from build123d import *

# Parameters (mm, degrees)
SKETCH1_R                  = 54.76875
BOSS_EXTRUDE1_DEPTH        = 6.35
BOSS_EXTRUDE2_START        = -6.35
BOSS_EXTRUDE2_DEPTH        = 6.35
F_1_0_228_DIAMETER_HOLE1_D = 5.7912
SKETCH11_R                 = 1.5875
CUT_EXTRUDE1_DEPTH         = 3.175
SKETCH12_R                 = 23.8125
CUT_EXTRUDE2_DEPTH         = 92.146558235


with BuildPart() as part:
    # Sketch1 → Boss-Extrude1 (new body)
    with BuildSketch(Plane.XY):
        Circle(SKETCH1_R)
    extrude(amount=BOSS_EXTRUDE1_DEPTH)

    # Sketch7 → Boss-Extrude2 (add)
    with BuildSketch(Plane.XY.offset(6.35).offset(BOSS_EXTRUDE2_START)):
        with BuildLine():
            Line((-54.561291868, 4.7625), (-59.53125, 4.7625))
            ThreePointArc((-59.53125, 4.7625), (-64.29375, 0), (-59.53125, -4.7625))
            Line((-59.53125, -4.7625), (-54.561291868, -4.7625))
            ThreePointArc((-54.561291868, -4.7625), (-54.76875, 0), (-54.561291868, 4.7625))
        make_face()
        with BuildLine():
            Line((-4.7625, 59.53125), (-4.7625, 54.561291868))
            ThreePointArc((-4.7625, 54.561291868), (0, 54.76875), (4.7625, 54.561291868))
            Line((4.7625, 54.561291868), (4.7625, 59.53125))
            ThreePointArc((4.7625, 59.53125), (0, 64.29375), (-4.7625, 59.53125))
        make_face()
        with BuildLine():
            ThreePointArc((4.7625, -54.561291868), (0, -54.76875), (-4.7625, -54.561291868))
            Line((-4.7625, -54.561291868), (-4.7625, -59.53125))
            ThreePointArc((-4.7625, -59.53125), (0, -64.29375), (4.7625, -59.53125))
            Line((4.7625, -59.53125), (4.7625, -54.561291868))
        make_face()
        with BuildLine():
            Line((59.53125, 4.7625), (54.561291868, 4.7625))
            ThreePointArc((54.561291868, 4.7625), (54.76875, 0), (54.561291868, -4.7625))
            Line((54.561291868, -4.7625), (59.53125, -4.7625))
            ThreePointArc((59.53125, -4.7625), (64.29375, 0), (59.53125, 4.7625))
        make_face()
    extrude(amount=BOSS_EXTRUDE2_DEPTH)

    # #1 (0.228) Diameter Hole1 (through all)
    with Locations(Plane.XY.offset(6.35)):
        with Locations((-59.53125, 0), (0, 59.53125), (59.53125, 0), (0, -59.53125)):
            Hole(F_1_0_228_DIAMETER_HOLE1_D / 2)

    # Sketch11 → Cut-Extrude1 (cut)
    with BuildSketch(Plane.XY.offset(6.35)):
        with Locations((-47.625, 0)):
            Circle(SKETCH11_R)
        with Locations((-46.584279485, 9.901794275)):
            Circle(SKETCH11_R)
        with Locations((-43.50760242, 19.370832626)):
            Circle(SKETCH11_R)
        with Locations((-38.529434357, 27.99327264)):
            Circle(SKETCH11_R)
        with Locations((-31.867345128, 35.392272313)):
            Circle(SKETCH11_R)
        with Locations((-23.8125, 41.244459855)):
            Circle(SKETCH11_R)
        with Locations((-14.716934357, 45.294066589)):
            Circle(SKETCH11_R)
        with Locations((-4.978168063, 47.364105267)):
            Circle(SKETCH11_R)
        with Locations((4.978168063, 47.364105267)):
            Circle(SKETCH11_R)
        with Locations((14.716934357, 45.294066589)):
            Circle(SKETCH11_R)
        with Locations((23.8125, 41.244459855)):
            Circle(SKETCH11_R)
        with Locations((31.867345128, 35.392272313)):
            Circle(SKETCH11_R)
        with Locations((38.529434357, 27.99327264)):
            Circle(SKETCH11_R)
        with Locations((43.50760242, 19.370832626)):
            Circle(SKETCH11_R)
        with Locations((46.584279485, 9.901794275)):
            Circle(SKETCH11_R)
        with Locations((47.625, 0)):
            Circle(SKETCH11_R)
        with Locations((46.584279485, -9.901794275)):
            Circle(SKETCH11_R)
        with Locations((43.50760242, -19.370832626)):
            Circle(SKETCH11_R)
        with Locations((38.529434357, -27.99327264)):
            Circle(SKETCH11_R)
        with Locations((31.867345128, -35.392272313)):
            Circle(SKETCH11_R)
        with Locations((23.8125, -41.244459855)):
            Circle(SKETCH11_R)
        with Locations((14.716934357, -45.294066589)):
            Circle(SKETCH11_R)
        with Locations((4.978168063, -47.364105267)):
            Circle(SKETCH11_R)
        with Locations((-4.978168063, -47.364105267)):
            Circle(SKETCH11_R)
        with Locations((-14.716934357, -45.294066589)):
            Circle(SKETCH11_R)
        with Locations((-23.8125, -41.244459855)):
            Circle(SKETCH11_R)
        with Locations((-31.867345128, -35.392272313)):
            Circle(SKETCH11_R)
        with Locations((-38.529434357, -27.99327264)):
            Circle(SKETCH11_R)
        with Locations((-43.50760242, -19.370832626)):
            Circle(SKETCH11_R)
        with Locations((-46.584279485, -9.901794275)):
            Circle(SKETCH11_R)
    extrude(amount=-CUT_EXTRUDE1_DEPTH, mode=Mode.SUBTRACT)

    # Sketch12 → Cut-Extrude2 (cut, through all)
    with BuildSketch(Plane.XY.offset(6.35)):
        Circle(SKETCH12_R)
    extrude(amount=-CUT_EXTRUDE2_DEPTH, mode=Mode.SUBTRACT)


solid = part.part
Design review of the part built by this model. Coordinates are the model's own, in mm. A direction names the side the tool comes from. Coordinates: 2 decimals unless noted, no trailing zeros. Order: outer loops, then holes, each group sorted by start corner. A loop starts at its lowest first (then second) coordinate and runs counter-clockwise, first axis right, second up.
Item 1: Take a section at C-C, the plane z = 1. Write out the cut boundary in (x, y) (1 decimal), then the cut area to 3 significant figures.
Item 2: Take a section at B-B, the plane x = 0. Write out the cut boundary in (y, z).
Item 3: Take a section at D-D, the plane x = -20. Write out the cut boundary in (y, z), then the cut area to 3 significant figures.
Item 4: For faces 1 (the flat face through (-57, 4.762, 3)), 2 (the cylindrical face through (-18.897, -14.49, 3.219)), 3 (the cylindrical face through (-5.18, 48.94, 4.78)), 4 (the flat face through (-57, -4.762, 3)), list the 3-axis set-ups (+Z, -Z, +X, -X, +Y, -Y) from which the entire face can be reached by the end or side of a thin tool; tool diameter is ignored.
Item 5: For line 1 (X direction, y = -19.5, z = 4.75); line 2 (X direction, y = -46, z = 4.5); line 3 (Y direction, x = -5.5, z = 5.5), list the stretches that pass through material, from the lowest coordinate up.
Item 6: For pin 1 Ø2 at (y, z) = (46.5, 1.5) entering from -X; pin 2 Ø1 at (x, z) = (13, 2.5) entering from +Y; pin 3 Ø1 at (x, z) = (32.5, 4.5) entering from -Y, all flat-tipped, find the tip position at first contact; note any pin that passes through.
Item 7: The part is to be moulded in two halves that separate along X. For faces 5 (the cylindrical face through (25.28, 40.64, 4.78)), 6 (the cylindrical face through (-39.1, -38.35, 3.13)), 7 (the flat face through (28, 1, 6.35)), say which applies: pulls with the +X half, pulls with the -X half, needs draft (parallel to the pull), parting line crosses it, or undercut.
Item 8: Take a section at A-A, the plane y = 0. Count the separate pieces of the cut face and the enclosed holes in it, then the cut area to 3 significant figures.
The answers:
1. outline: (-59.5, -4.8) - (-54.6, -4.8) arc R54.8 ccw to (-4.8, -54.6) - (-4.8, -59.5) arc R4.8 ccw to (4.8, -59.5) - (4.8, -54.6) arc R54.8 ccw to (54.6, -4.8) - (59.5, -4.8) arc R4.8 ccw to (59.5, 4.8) - (54.6, 4.8) arc R54.8 ccw to (4.8, 54.6) - (4.8, 59.5) arc R4.8 ccw to (-4.8, 59.5) - (-4.8, 54.6) arc R54.8 ccw to (-54.6, 4.8) - (-59.5, 4.8) arc R4.8 ccw to start; hole circle Ø5.8 at (-59.5, 0); hole circle Ø47.6 at (0, 0); hole circle Ø5.8 at (0, -59.5); hole circle Ø5.8 at (0, 59.5); hole circle Ø5.8 at (59.5, 0)
1. area: 7,860 mm2
2. outline: (-64.29, 0) - (-62.43, 0) - (-62.43, 6.35) - (-64.29, 6.35) - close; (-56.64, 0) - (-23.81, 0) - (-23.81, 6.35) - (-56.64, 6.35) - close; (23.81, 0) - (56.64, 0) - (56.64, 6.35) - (23.81, 6.35) - close; (62.43, 0) - (64.29, 0) - (64.29, 6.35) - (62.43, 6.35) - close
3. outline: (-50.99, 0) - (-12.92, 0) - (-12.92, 6.35) - (-50.99, 6.35) - close; (12.92, 0) - (50.99, 0) - (50.99, 6.35) - (12.92, 6.35) - close
3. area: 483 mm2
4. face 1: +Z, -Z, -X, +Y
4. face 2: +Z, -Z
4. face 3: +Z
4. face 4: +Z, -Z, -X, -Y
5. line 1: x = -51.18 to -45.09, -41.93 to -13.67, 13.67 to 41.93, 45.09 to 51.18
5. line 2: x = -29.73 to -16.14, -13.3 to -5.79, -4.17 to 4.17, 5.79 to 13.3, 16.14 to 29.73
5. line 3: y = -54.49 to -48.86, -45.86 to -23.17, 23.17 to 45.86, 48.86 to 54.49
6. pin 1: stops at x = -30.49
6. pin 2: stops at y = 53.32
6. pin 3: stops at y = -44.45
7. face 5: undercut
7. face 6: pulls with the -X half
7. face 7: needs draft
8. separate pieces: 4
8. enclosed holes: 0
8. area: 420 mm2
